from build123d import *

# Parameters (mm, degrees)
F0_R      = 12.5
F1_DEPTH  = 3
F1_FACE_R = 12.5
F2_DEPTH  = 0.5
F2_TAPER  = 45
F2_FACE_R = 12
F3_DEPTH  = 2.5
F3_TAPER  = -10
F3_FACE_R = 12.4408174518
F4_DEPTH  = 2
F4_TAPER  = 30
F4_FACE_R = 11.2861169134
F5_DEPTH  = 3
F5_TAPER  = 35
F5_FACE_R = 9.1854942988
F6_DEPTH  = 1.5
F6_TAPER  = -45
F6_FACE_R = 10.6854942988
F7_DEPTH  = 1.5
F7_TAPER  = 60
F7_FACE_R = 8.0874180874
F8_DEPTH  = 10
F8_TAPER  = 15
F8_FACE_R = 5.4079261631
F9_DEPTH  = 2
F9_TAPER  = -45
F9_FACE_R = 7.4079261631
F10_DEPTH = 1
F10_TAPER = 60


with BuildPart() as f1:
    # F0 (on Top) → F1 (new body)
    with BuildSketch(Plane.XY):
        Circle(F0_R)
    extrude(amount=F1_DEPTH)

    # F1_face (on face) → F2 (join)
    with BuildSketch(Plane.XY.offset(3)):
        Circle(F1_FACE_R)
    extrude(amount=F2_DEPTH, taper=F2_TAPER)

    # F2_face (on face) → F3 (join)
    with BuildSketch(Plane.XY.offset(3.5)):
        Circle(F2_FACE_R)
    extrude(amount=F3_DEPTH, taper=F3_TAPER)

    # F3_face (on face) → F4 (join)
    with BuildSketch(Plane.XY.offset(6)):
        Circle(F3_FACE_R)
    extrude(amount=F4_DEPTH, taper=F4_TAPER)

    # F4_face (on face) → F5 (join)
    with BuildSketch(Plane.XY.offset(8)):
        Circle(F4_FACE_R)
    extrude(amount=F5_DEPTH, taper=F5_TAPER)

    # F5_face (on face) → F6 (join)
    with BuildSketch(Plane.XY.offset(11)):
        Circle(F5_FACE_R)
    extrude(amount=F6_DEPTH, taper=F6_TAPER)

    # F6_face (on face) → F7 (join)
    with BuildSketch(Plane.XY.offset(12.5)):
        Circle(F6_FACE_R)
    extrude(amount=F7_DEPTH, taper=F7_TAPER)

    # F7_face (on face) → F8 (join)
    with BuildSketch(Plane.XY.offset(14)):
        Circle(F7_FACE_R)
    extrude(amount=F8_DEPTH, taper=F8_TAPER)

    # F8_face (on face) → F9 (join)
    with BuildSketch(Plane.XY.offset(24)):
        Circle(F8_FACE_R)
    extrude(amount=F9_DEPTH, taper=F9_TAPER)

    # F9_face (on face) → F10 (join)
    with BuildSketch(Plane.XY.offset(26)):
        Circle(F9_FACE_R)
    extrude(amount=F10_DEPTH, taper=F10_TAPER)

    # F11 (on Front) → F12 (revolve)
    with BuildSketch(Plane.XZ):
        with BuildLine():
            ThreePointArc((0, 40), (-7.5, 32.5), (0, 25))
            Line((0, 25), (0, 40))
        make_face()
    revolve(axis=Axis((0, 0, 21.0038799897), (0, 0, 1)))


solid = f1.part
Verification items for the finished model (mm, model axes). Give positions to 0.01 mm unless a question says otherwise; leave off trailing zeros. Write each loop counter-clockwise with the first axis right and the second up, starting at its lowest first coordinate (ties: lowest second). Pieces come first, ordered by that corner, then holes. Notation, with made-up numbers: (9.25, -20.75) -> (51.25, -20.75) arc R13 cw to (51.25, -14.75) -> close; hole circle Ø11 at (-11.5, 45). An arc over 180 degrees is marked (long way). Use CSV: the item, a comma, the result in double quotes.
(1) Sectioned sample at A-A (x = 0). Record the cut outline in (y, z), plus the area to 3 significant figures.
Derived:
outline,"(-12.5, 0) -> (12.5, 0) -> (12.5, 3) -> (12, 3.5) -> (12.44, 6) -> (11.29, 8) -> (9.19, 11) -> (10.69, 12.5) -> (8.09, 14) -> (5.41, 24) -> (7.41, 26) -> (5.68, 27) -> (5.1, 27) arc R7.5 ccw (long way) to (-5.1, 27) -> (-5.68, 27) -> (-7.41, 26) -> (-5.41, 24) -> (-8.09, 14) -> (-10.69, 12.5) -> (-9.19, 11) -> (-11.29, 8) -> (-12.44, 6) -> (-12, 3.5) -> (-12.5, 3) -> close"
area,"652 mm^2"
(2) Sectioned sample at B-B (z = 11.5). Record the cut outline in (x, y).
Derived:
outline,"circle Ø19.37 at (0, 0)"
(3) Material ranges on L1, parallel to Z at x = 1.5, y = 9.75; L2, parallel to Z at x = 0, y = 10.25; L3, parallel to Z at x = -8, y = 4.25, recorded low to high.
Derived:
L1,"z = 0 to 10.03, 11.68 to 12.97"
L2,"z = 0 to 9.48, 12.06 to 12.75"
L3,"z = 0 to 13.44"
(4) Sectioned sample at C-C (z = 30.5). Record the cut outline in (x, y), plus the area to 3 significant figures.
Derived:
outline,"circle Ø14.46 at (0, 0)"
area,"164 mm^2"
(5) Release check for a two-part mould opening along Z. For faces 1 (the conical face through (-1.199, -5.401, 24.125)), 2 (the flat face through (0, 0, 0)), 3 (the cylindrical face through (11.923, 3.755, 1.479)) record: +Z half, -Z half, draft (parallel to the pull), parting line (faces both ways), or undercut.
Derived:
face 1,"undercut"
face 2,"-Z half"
face 3,"draft"
(6) Go/stop test with flat-tipped pins: pin 1 (4 mm diameter, centred on x = 9, y = 0.5, fed in from -Z); pin 2 (2 mm diameter, centred on y = 10, z = 5, fed in from -X); pin 3 (10 mm diameter, centred on x = 3.5, z = 19.5, fed in from -Y); pin 4 (12 mm diameter, centred on y = 2.5, z = 24.5, fed in from -X). Record where each tip stops, or that it passes through.
Derived:
pin 1,"stops at z = 0"
pin 2,"stops at x = -8.36"
pin 3,"stops at y = -7.71"
pin 4,"stops at x = -7.41"
